Geometry check sheet. Reference: drawing and pictorial views, mm from the part's lowest x, y, z. A direction names the side the tool comes from. Give positions to 0.01 mm unless a question says otherwise; leave off trailing zeros. Order: outer loops, then holes, each group sorted by start corner. A loop starts at its lowest first (then second) coordinate and runs counter-clockwise, first axis right, second up. Notation, with made-up numbers: (-18, -18) - (-8, -18) arc R21 cw to (-8, -9) - close; hole circle Ø7 at (50, 64.25). An arc over 180 degrees is marked (long way). Answer as a JSON object with one key per item and string values.
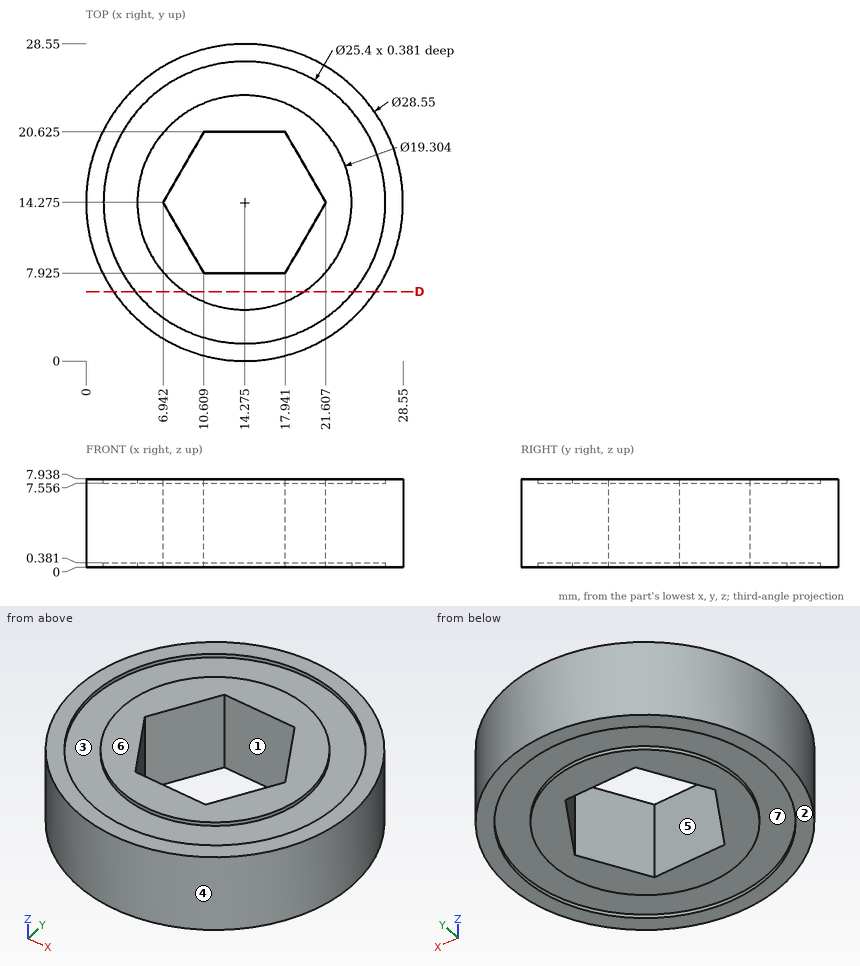
(1) Material ranges on line 1 along Z through (x, y) = (16.25, 26.5); line 2 along X through (y, z) = (16.5, 3.5) (1 decimal); line 3 along Y through (x, z) = (18.25, 5) (1 decimal), recorded low to high. Write a range as [from, to].
Computed values:
{"line 1": "z = [0.38, 7.56]", "line 2": "x = [0.2, 8.2], [20.3, 28.4]", "line 3": "y = [0.6, 8.5], [20.1, 28]"}
(2) Gauge pin test, flat ends, axial feed: pin 1 Ø2 at (x, z) = (12.5, 5) entering from +Y; pin 2 Ø4 at (y, z) = (9, 7) entering from -X; pin 3 Ø4 at (y, z) = (16.5, 7) entering from +X. Record the tip position at first contact, or that the pin passes through.
Computed values:
{"pin 1": "stops at y = 28.53", "pin 2": "stops at x = 0.38", "pin 3": "stops at x = 28.55"}
(3) Access from +Z, -Z, +X, -X, +Y, -Y to the whole of each face (thin tool, end or side, straight path). Record for the marked faces 1, 2 and 3.
Computed values:
{"face 1": "+Z, -Z", "face 2": "-Z, +X, -X, +Y, -Y", "face 3": "+Z"}
(4) Section check D-D (y = 6.25). Record the cut outline in (x, z).
Computed values:
{"outline": "(2.47, 0) - (4.43, 0) - (4.43, 0.38) - (8.91, 0.38) - (8.91, 0) - (19.64, 0) - (19.64, 0.38) - (24.12, 0.38) - (24.12, 0) - (26.08, 0) - (26.08, 7.94) - (24.12, 7.94) - (24.12, 7.56) - (19.64, 7.56) - (19.64, 7.94) - (8.91, 7.94) - (8.91, 7.56) - (4.43, 7.56) - (4.43, 7.94) - (2.47, 7.94) - close"}
(5) Release check for a two-part mould opening along X. For the marked faces 4, 5, 6 and 7 record: pulls with the +X half, pulls with the -X half, needs draft (parallel to the pull), parting line crosses it, or undercut.
Computed values:
{"face 4": "parting line crosses it", "face 5": "undercut", "face 6": "needs draft", "face 7": "undercut"}
